Work out the finished part from the listing and answer in its coordinate system (mm). Face numbers are marked on the shaded views. A direction names the side the tool comes from. Round coordinates to 2 decimals unless told otherwise and drop trailing zeros. Write each loop counter-clockwise with the first axis right and the second up, starting at its lowest first coordinate (ties: lowest second). Pieces come first, ordered by that corner, then holes. Notation, with made-up numbers: (20, -13) -> (63, -13) arc R18 cw to (63, 5) -> close; hole circle Ø6 at (54, 27). An arc over 180 degrees is marked (long way). One line per item, written item: value.
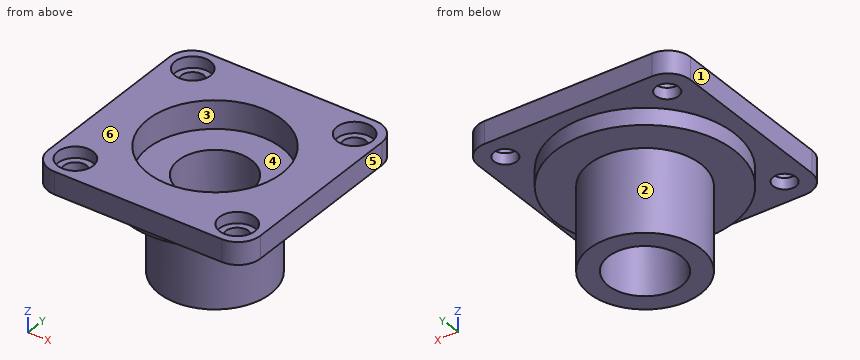
Solid Edge part; units mm, degrees
sketch "Sketch1" plane through (0, 0, 0) normal (0, 0, 1) x (1, 0, 0)
  line L0 (15, 19) -> (-15, 19)
  arc A0 (-15, 19) -> (-19, 15) centre (-15, 15) ccw
  line L1 (-19, 15) -> (-19, -15)
  arc A1 (-19, -15) -> (-15, -19) centre (-15, -15) ccw
  line L2 (-15, -19) -> (15, -19)
  arc A2 (15, -19) -> (19, -15) centre (15, -15) ccw
  line L3 (19, -15) -> (19, 15)
  arc A3 (15, 19) -> (19, 15) centre (15, 15) cw
extrude "Protrusion1" add sketch "Sketch1" along normal blind 4
sketch "Sketch2" plane through (0, 0, 0) normal (0, 0, -1) x (-1, 0, 0)
  circle A0 centre (0, 0) radius 16
extrude "Protrusion2" add sketch "Sketch2" along normal blind 3
sketch "Sketch3" plane through (0, 0, -3) normal (0, 0, -1) x (-1, 0, 0)
  circle A0 centre (0, 0) radius 10
extrude "Protrusion3" add sketch "Sketch3" along normal blind 14.8
sketch "Sketch4" plane through (0, 0, 4) normal (0, 0, 1) x (1, 0, 0)
  circle A0 centre (0, 0) radius 12
extrude "Cutout1" cut sketch "Sketch4" against normal blind 5
sketch "Sketch5" plane through (0, 0, -1) normal (0, 0, 1) x (1, 0, 0)
  circle A0 centre (0, 0) radius 6.55
extrude "Cutout2" cut sketch "Sketch5" against normal up to next
hole "Hole_1" at (-14.5, 14.5, 4) direction (0, 0, -1) diameter 4.1 end up to next counterbore diameter 6.35 counterbore depth 2
hole "Hole1" at (14.5, 14.5, 4) direction (0, 0, -1) diameter 4.1 end up to next counterbore diameter 6.35 counterbore depth 2
hole "Hole_3" at (14.5, -14.5, 4) direction (0, 0, -1) diameter 4.1 end up to next counterbore diameter 6.35 counterbore depth 2
hole "Hole_4" at (-14.5, -14.5, 4) direction (0, 0, -1) diameter 4.1 end up to next counterbore diameter 6.35 counterbore depth 2
properties part number "PLATE1" material "410 Stainless Steel"
(1) Consider probe 1 along X at (y, z) = (14.5, 1.3); probe 2 along Y at (x, z) = (14.5, 3.2) (3 decimals). Determine where each line is inside the solid, lowest interval first.
Reported:
probe 1: x = -19 to -16.55, -12.45 to 12.45, 16.55 to 19
probe 2: y = -19 to -17.675, -11.325 to 11.325, 17.675 to 19
(2) A tool of negligible diameter and unlimited length cuts with its end or side. For the marked faces 1, 2 and 3, from which of +Z, -Z, +X, -X, +Y, -Y can it reach the whole face along a straight path? Write none if from no direction.
Reported:
face 1: +Z, -Z, -X, +Y, -Y
face 2: -Z
face 3: +Z
(3) Find section A-A on x = 0. Give the vertices of the cut face in (y, z).
Reported:
outline: (-19, 0) -> (-16, 0) -> (-16, -3) -> (-10, -3) -> (-10, -17.8) -> (-6.55, -17.8) -> (-6.55, -1) -> (-12, -1) -> (-12, 4) -> (-19, 4) -> close; (6.55, -17.8) -> (10, -17.8) -> (10, -3) -> (16, -3) -> (16, 0) -> (19, 0) -> (19, 4) -> (12, 4) -> (12, -1) -> (6.55, -1) -> close
(4) Find section D-D on x = 15.5. Give the vertices of the cut face in (y, z), plus the area to 3 significant figures.
Reported:
outline: (-18.97, 0) -> (-16.29, 0) -> (-16.29, 2) -> (-17.51, 2) -> (-17.51, 4) -> (-18.97, 4) -> close; (-12.71, 0) -> (-3.97, 0) -> (-3.97, -3) -> (3.97, -3) -> (3.97, 0) -> (12.71, 0) -> (12.71, 2) -> (11.49, 2) -> (11.49, 4) -> (-11.49, 4) -> (-11.49, 2) -> (-12.71, 2) -> close; (16.29, 0) -> (18.97, 0) -> (18.97, 4) -> (17.51, 4) -> (17.51, 2) -> (16.29, 2) -> close
area: 137 mm2
(5) Find section B-B on y = -6. Give the vertices of the cut face in (x, z), plus the area to 3 significant figures.
Reported:
outline: (-19, 0) -> (-14.83, 0) -> (-14.83, -3) -> (-8, -3) -> (-8, -17.8) -> (-2.63, -17.8) -> (-2.63, -1) -> (-10.39, -1) -> (-10.39, 4) -> (-19, 4) -> close; (2.63, -17.8) -> (8, -17.8) -> (8, -3) -> (14.83, -3) -> (14.83, 0) -> (19, 0) -> (19, 4) -> (10.39, 4) -> (10.39, -1) -> (2.63, -1) -> close
area: 286 mm2
(6) For a pull along X with two mould halves and no side action, classify the marked faces 4, 5 and 6 as pulls with the +X half, pulls with the -X half, needs draft (parallel to the pull), parting line crosses it, or undercut.
Reported:
face 4: undercut
face 5: pulls with the +X half
face 6: needs draft
(7) Find section C-C on z = 1.25. Give the vertices of the cut face in (x, y), plus the area to 3 significant figures.
Reported:
outline: (-19, -15) arc R4 ccw to (-15, -19) -> (15, -19) arc R4 ccw to (19, -15) -> (19, 15) arc R4 ccw to (15, 19) -> (-15, 19) arc R4 ccw to (-19, 15) -> close; hole circle Ø4.1 at (-14.5, -14.5); hole circle Ø4.1 at (-14.5, 14.5); hole circle Ø24 at (0, 0); hole circle Ø4.1 at (14.5, -14.5); hole circle Ø4.1 at (14.5, 14.5)
area: 925 mm2
(8) Flat-ended cylindrical pins translate along their axes: pin 1 Ø5 at (x, z) = (-13, -14) entering from -Y; pin 2 Ø5.5 at (x, y) = (14.5, -14.5) entering from +Z; pin 3 Ø21.5 at (x, y) = (0, 0) entering from -Z; pin 4 Ø12 at (x, z) = (-4.5, -8.5) entering from +Y. Find the tip coordinate at first contact, or state that the pin passes through.
Reported:
pin 1: passes through
pin 2: stops at z = 2
pin 3: stops at z = -17.8
pin 4: stops at y = 15.86
